Could you check a few things on this drawing? It's one solid part, dimensions in mm from its lowest x, y, z. Coordinates: 2 decimals unless noted, no trailing zeros. Loops run counter-clockwise (first coordinate to the right, second up) from the corner with the lowest first, then second, coordinate; pieces in that order, holes last. Notation, with made-up numbers: (28.25, 29.25) -> (73.25, 29.25) arc R17 ccw to (73.25, 37.25) -> close; hole circle Ø9 at (49, -22.5). An arc over 180 degrees is marked (long way). One line per question, with ' | ' between items. Start each with the question number.
(1) I'm going to push flat-ended pins straight in: pin 1 Ø2 at (x, y) = (10.5, 70) entering from +Z; pin 2 Ø1.5 at (x, y) = (29, 134) entering from -Z; pin 3 Ø5.5 at (x, z) = (30, 10) entering from -Y. Where does each tip first touch, or does it pass through?
(2) Suppose I cut it at C-C (y = 155.5). Please give me the cut outline in (x, z).
(3) If I drill on line 1 along X through (y, z) = (65.5, 18); line 2 along X through (y, z) = (35, 9.25); line 3 along Z through (x, y) = (30, 130), over which ranges is the centre line in solid material (lowest first)?
(4) Suppose I cut it at A-A (x = 10). Please give me the cut outline in (y, z), plus the area to 4 significant figures.
(5) Suppose I cut it at B-B (z = 10). Please give me the cut outline in (x, y).
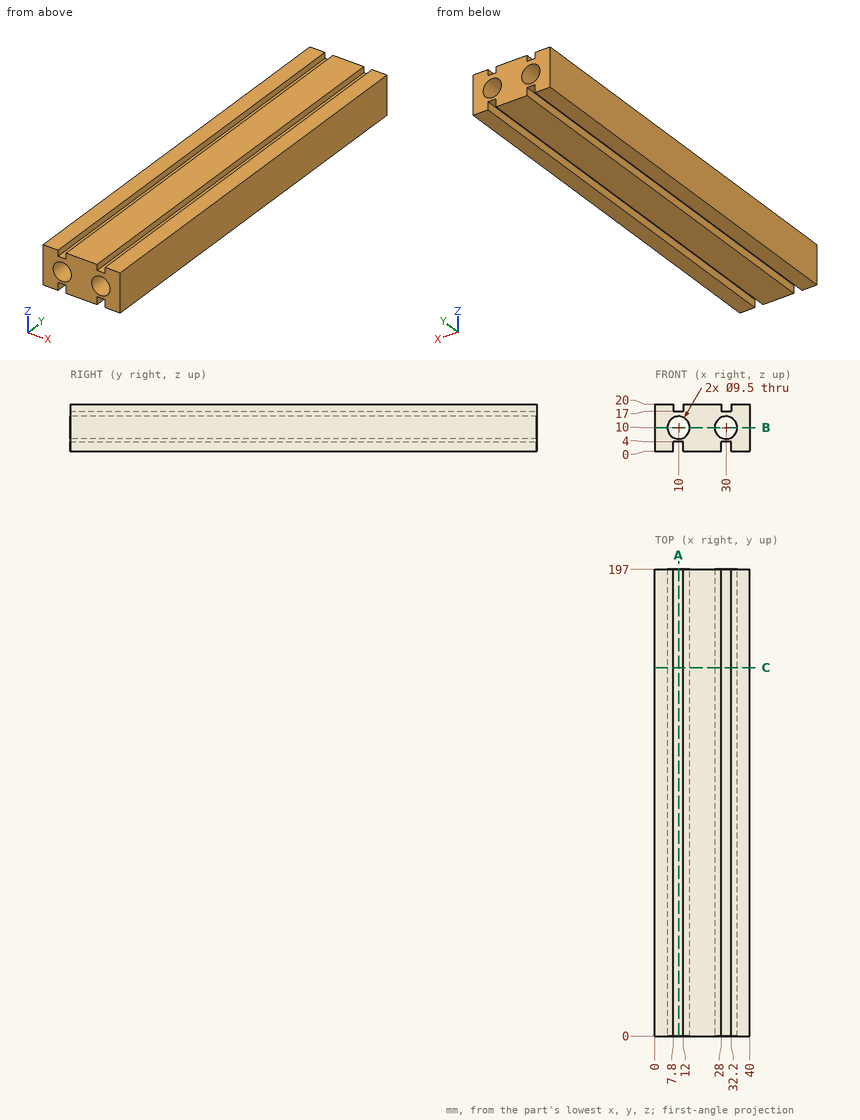
Checks:
1) pin 1: stops at z = 17 | pin 2: stops at z = 4 | pin 3: passes through
2) outline: (0, 0) -> (7.8, 0) -> (7.8, 4) -> (12, 4) -> (12, 0) -> (28, 0) -> (28, 4) -> (32.2, 4) -> (32.2, 0) -> (40, 0) -> (40, 20) -> (32.2, 20) -> (32.2, 17) -> (28, 17) -> (28, 20) -> (12, 20) -> (12, 17) -> (7.8, 17) -> (7.8, 20) -> (0, 20) -> close; hole circle Ø9.5 at (10, 10); hole circle Ø9.5 at (30, 10)
3) line 1: x = 0 to 7.8, 12 to 28, 32.2 to 40 | line 2: x = 0 to 5.31, 14.69 to 25.31, 34.69 to 40 | line 3: z = 4 to 5.25, 14.75 to 17
4) outline: (0, 4) -> (197, 4) -> (197, 5.25) -> (0, 5.25) -> close; (0, 14.75) -> (197, 14.75) -> (197, 17) -> (0, 17) -> close | area: 689.5 mm^2
5) outline: (0, 0) -> (5.25, 0) -> (5.25, 197) -> (0, 197) -> close; (14.75, 0) -> (25.25, 0) -> (25.25, 197) -> (14.75, 197) -> close; (34.75, 0) -> (40, 0) -> (40, 197) -> (34.75, 197) -> close
